Here's how the part is built. I have some questions about the finished solid (model axes, mm). Face numbers are marked on the shaded views. A direction names the side the tool comes from. Coordinates: 2 decimals unless noted, no trailing zeros. Write each loop counter-clockwise with the first axis right and the second up, starting at its lowest first coordinate (ties: lowest second). Pieces come first, ordered by that corner, then holes.
(1) Imagine slicing it at B-B, the plane x = -40. List the corners of the cut face in (y, z) for me, plus the area to 3 significant figures.
(2) Imagine slicing it at C-C, the plane z = 252. List the corners of the cut face in (x, y) for me.
(3) Thinking about a two-plate mould opening in Y: for the marked faces 1, 2 and 3, which applies, released by +Y, released by -Y, zero draft, split by the parting line, or undercut?
(4) Please list where these lines run through material, in increasing order: probe 1 along Z at (x, y) = (0, 57.2); probe 2 along Y at (x, z) = (36, 206); probe 3 along Y at (x, z) = (7.5, 169).
(5) Imagine slicing it at A-A, the plane y = -40. List the corners of the cut face in (x, z) for me, plus the area to 3 significant figures.
(6) For pin 1 Ø2.5 at (x, y) = (16, -57) entering from +Z; pin 2 Ø4 at (x, y) = (-25.5, -26.5) entering from +Z; pin 3 Ø2.5 at (y, z) = (-57.5, 192) entering from +X, each with a flat end and sliding along its axis, tell me the tip position at first contact or that it passes through.
(7) Which directions (+Z, -Z, +X, -X, +Y, -Y) give clear straight access to the entire face, cutting with the end or side of a thin tool? Please do the marked faces 4 and 5.
(8) Imagine slicing it at D-D, the plane y = 0. List the corners of the cut face in (x, z) for me, plus the area to 3 significant figures.
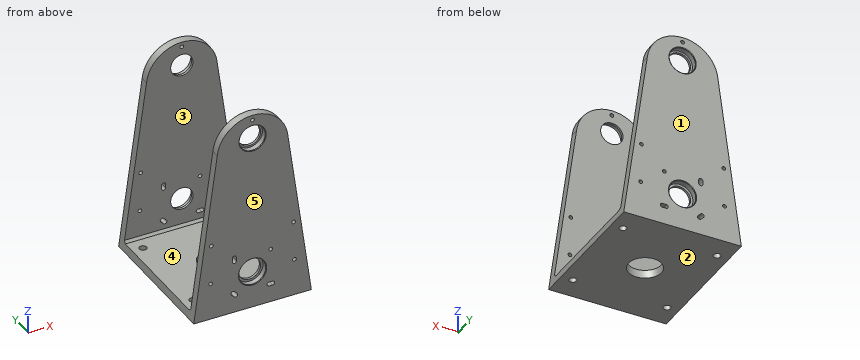
```python
from build123d import *

# Parameters (mm, degrees)
SKETCH155_R             = 9.5
SKETCH155_R_2           = 1.6
PAD044_DEPTH            = 120
POCKET098_DEPTH         = 152.4
SKETCH152_R             = 3.1
SKETCH152_R_2           = 14
POCKET096_DEPTH         = 8
SKETCH156_R             = 1.575
POCKET099_DEPTH         = 120
SKETCH157_R             = 11.5
SKETCH157_R_2           = 11.1
POCKET100_DEPTH         = 5
SKETCH158_R             = 11.1
SKETCH158_R_2           = 11.5
POCKET101_DEPTH         = 5
CHAMFER026_SIZE         = 0.5
BODY034_PLACEMENT_ANGLE = 90


with BuildPart() as part:
    # Sketch155 → Pad044 (new body)
    with BuildSketch(Plane.XY):
        with BuildLine():
            Line((-50, 70), (50, 70))
            Line((50, 70), (30, 215))
            ThreePointArc((30, 215), (0, 242.2218283079), (-30, 215))
            Line((-50, 70), (-30, 215))
        make_face()
        with Locations((0, 221.5800627023)):
            Circle(SKETCH155_R, mode=Mode.SUBTRACT)
        with Locations((0, 101.5800627023)):
            Circle(SKETCH155_R, mode=Mode.SUBTRACT)
        with Locations((-35.6441292824, 101.5800627023)):
            Circle(SKETCH155_R_2, mode=Mode.SUBTRACT)
        with Locations((35.6441292824, 101.5800627023)):
            Circle(SKETCH155_R_2, mode=Mode.SUBTRACT)
        with Locations((-34.9725747282, 135.4488332209)):
            Circle(SKETCH155_R_2, mode=Mode.SUBTRACT)
        with Locations((34.9725747282, 135.4488332209)):
            Circle(SKETCH155_R_2, mode=Mode.SUBTRACT)
        with Locations((0, 238)):
            Circle(SKETCH155_R_2, mode=Mode.SUBTRACT)
    extrude(amount=PAD044_DEPTH)

    # Sketch154 → Pocket098 (cut, symmetric)
    with BuildSketch(Plane(origin=(0, 0, 120), x_dir=(0, 0, -1), z_dir=(1, 0, 0))):
        Polygon((7, 252.37), (113, 252.37), (113, 79), (111, 77), (9, 77), (7, 79), align=None)
    extrude(amount=POCKET098_DEPTH, both=True, mode=Mode.SUBTRACT)

    # Sketch152 (on Face1 of Pocket098) → Pocket096 (cut)
    with BuildSketch(Plane.XZ.offset(-70)):
        with Locations((-40, 100)):
            Circle(SKETCH152_R)
        with Locations((40, 100)):
            Circle(SKETCH152_R)
        with Locations((-40, 20)):
            Circle(SKETCH152_R)
        with Locations((40, 20)):
            Circle(SKETCH152_R)
        with Locations((0, 60)):
            Circle(SKETCH152_R_2)
    extrude(amount=-POCKET096_DEPTH, mode=Mode.SUBTRACT)

    # Sketch156 → Pocket099 (cut)
    with BuildSketch(Plane.XY.offset(120)):
        with Locations((15.5, 117.0800628443)):
            Circle(SKETCH156_R)
        with BuildLine():
            ThreePointArc((-13.75, 118.6550628443), (-15.5, 120.4050628443), (-17.25, 118.6550628443))
            Line((-17.25, 118.6550628443), (-17.25, 115.5050628443))
            ThreePointArc((-17.25, 115.5050628443), (-15.5, 113.7550628443), (-13.75, 115.5050628443))
            Line((-13.75, 118.6550628443), (-13.75, 115.5050628443))
        make_face()
        with BuildLine():
            ThreePointArc((13.925, 87.8300628443), (12.175, 86.0800628443), (13.925, 84.3300628443))
            Line((13.925, 84.3300628443), (17.075, 84.3300628443))
            ThreePointArc((17.075, 84.3300628443), (18.825, 86.0800628443), (17.075, 87.8300628443))
            Line((13.925, 87.8300628443), (17.075, 87.8300628443))
        make_face()
        with BuildLine():
            ThreePointArc((-15.3762563133, 88.4311928917), (-17.8511300474, 88.4311928917), (-17.8511300474, 85.9563191575))
            Line((-17.8511300474, 85.9563191575), (-15.6237436867, 83.7289327968))
            ThreePointArc((-15.6237436867, 83.7289327968), (-13.1488699526, 83.7289327968), (-13.1488699525, 86.203806531))
            Line((-15.3762563133, 88.4311928917), (-13.1488699525, 86.203806531))
        make_face()
    extrude(amount=-POCKET099_DEPTH, mode=Mode.SUBTRACT)

    # Sketch157 (on Face3 of Pocket099) → Pocket100 (cut)
    with BuildSketch(Plane(origin=(0, 0, 0), x_dir=(1, 0, 0), z_dir=(0, 0, -1))):
        with Locations((0, -101.5800627023)):
            Circle(SKETCH157_R)
        with Locations((0, -221.5800627023)):
            Circle(SKETCH157_R_2)
    extrude(amount=-POCKET100_DEPTH, mode=Mode.SUBTRACT)

    # Sketch158 (on Face4 of Pocket100) → Pocket101 (cut)
    with BuildSketch(Plane.XY.offset(120)):
        with Locations((0, 221.5800627023)):
            Circle(SKETCH158_R)
        with Locations((0, 101.5800627023)):
            Circle(SKETCH158_R_2)
    extrude(amount=-POCKET101_DEPTH, mode=Mode.SUBTRACT)

    # Chamfer026
    chamfer026_edges = [part.edges().sort_by_distance(p)[0] for p in [
        (-11.1, 221.580063, 120),
        (-11.5, 101.580063, 120),
        (-11.1, 221.580063, 0),
        (-11.5, 101.580063, 0),
    ]]
    chamfer(chamfer026_edges, length=CHAMFER026_SIZE)


with BuildPart() as part_1:
    # Body034 placement: moved
    add(part.part.moved(Location((0, 60, 75.6))).rotate(Axis((0, 60, 75.6), (1, 0, 0)), BODY034_PLACEMENT_ANGLE))


solid = part_1.part
```
Recorded:
1. outline: (-60, 145.6) - (-43.1, 145.6) - (-43.1, 152.6) - (-51, 152.6) - (-53, 154.6) - (-53, 218.1) - (-60, 218.1) - close; (-36.9, 145.6) - (36.9, 145.6) - (36.9, 152.6) - (-36.9, 152.6) - close; (43.1, 145.6) - (60, 145.6) - (60, 218.1) - (53, 218.1) - (53, 154.6) - (51, 152.6) - (43.1, 152.6) - close
1. area: 1,670 mm2
2. outline: (-35.32, -60) - (35.32, -60) - (35.32, -53) - (-35.32, -53) - close; (-35.32, 53) - (35.32, 53) - (35.32, 60) - (-35.32, 60) - close
3. face 1: released by +Y
3. face 2: zero draft
3. face 3: undercut
4. probe 1: z = 145.6 to 165.68, 188.68 to 286.08, 308.28 to 312, 315.2 to 317.82
4. probe 2: y = -60 to -53, 53 to 60
4. probe 3: y = -55 to -53, 53 to 55
5. outline: (-50, 145.6) - (-43.1, 145.6) - (-43.1, 152.6) - (-49.03, 152.6) - close; (-36.9, 145.6) - (36.9, 145.6) - (36.9, 152.6) - (-36.9, 152.6) - close; (43.1, 145.6) - (50, 145.6) - (49.03, 152.6) - (43.1, 152.6) - close
5. area: 606 mm2
6. pin 1: stops at z = 313.97
6. pin 2: stops at z = 152.6
6. pin 3: stops at x = 43.77
7. face 4: +Z, +X, -X
7. face 5: +Z, -Z, +X, -X, -Y
8. outline: (-50, 145.6) - (-14, 145.6) - (-14, 152.6) - (-49.03, 152.6) - close; (14, 145.6) - (50, 145.6) - (49.03, 152.6) - (14, 152.6) - close
8. area: 497 mm2
